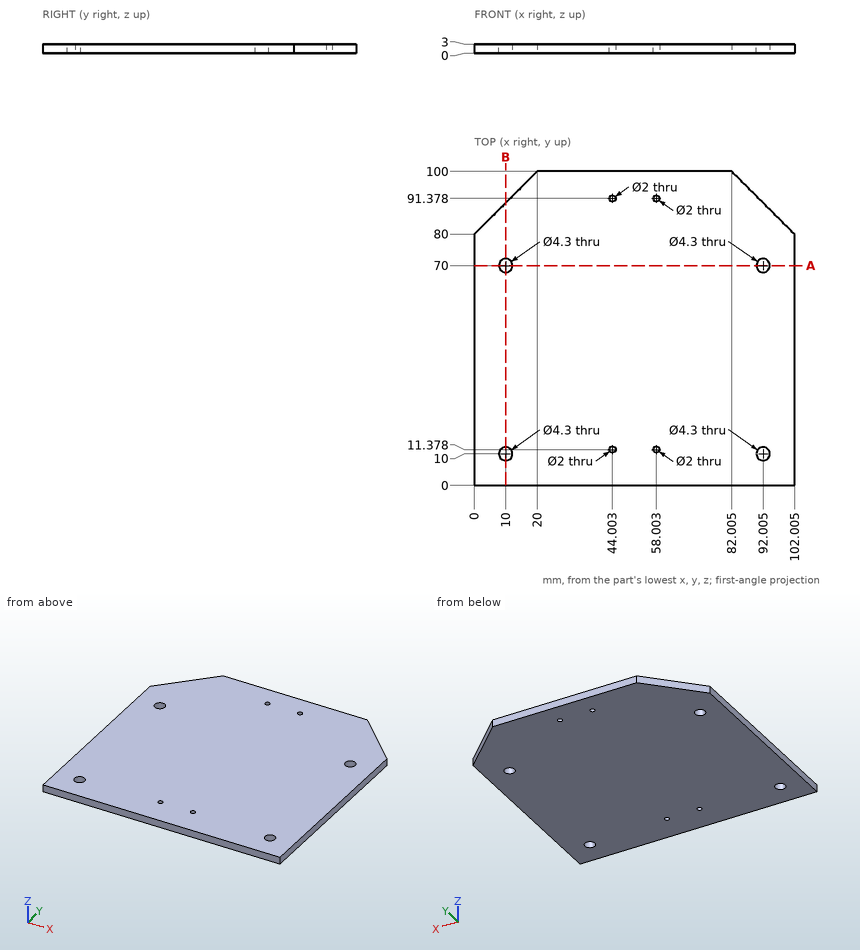
Drawing for the job (mm, zero at the part's lowest x, y, z). Round coordinates to 2 decimals unless told otherwise and drop trailing zeros. Write each loop counter-clockwise with the first axis right and the second up, starting at its lowest first coordinate (ties: lowest second). Pieces come first, ordered by that corner, then holes. Notation, with made-up numbers: (-5, -34.75) - (27, -34.75) arc R11 cw to (27, -29.75) - close; hole circle Ø9 at (59, 51). An arc over 180 degrees is marked (long way). Return JSON: item names as keys, results as strings. Group by question number.
Item 1: Flat gauge pin, fed straight in: pin 1 Ø1.5 at (y, z) = (59, 0.5) entering from -X. Where does the tip first touch, or does it go through?
Item 2: Probe probe 1 along Y at (x, z) = (10, 1.2); probe 2 along X at (y, z) = (69.5, 1.35) (1 decimal); probe 3 along X at (y, z) = (11, 2.7) (1 decimal). List the from-to ranges inside material, lowest first.
Item 3: Band-saw the part on B-B on x = 10. List the corners of the cut face in (y, z).
Item 4: Band-saw the part on A-A on y = 70. State how many separate pieces and enclosed holes the cut face has, plus the area to 3 significant figures.
Resolved:
{
 "1": {"pin 1": "stops at x = 0"},
 "2": {"probe 1": "y = 0 to 7.85, 12.15 to 67.85, 72.15 to 90", "probe 2": "x = 0 to 7.9, 12.1 to 89.9, 94.1 to 102", "probe 3": "x = 0 to 8.1, 11.9 to 43.1, 44.9 to 57.1, 58.9 to 90.1, 93.9 to 102"},
 "3": {"outline": "(0, 0) - (7.85, 0) - (7.85, 3) - (0, 3) - close; (12.15, 0) - (67.85, 0) - (67.85, 3) - (12.15, 3) - close; (72.15, 0) - (90, 0) - (90, 3) - (72.15, 3) - close"},
 "4": {"separate pieces": "3", "enclosed holes": "0", "area": "280 mm²"}
}
